```python
from build123d import *

# Parameters (mm, degrees)
PAD005_DEPTH    = 2
SKETCH011_W     = 2
SKETCH011_H     = 6
PAD006_DEPTH    = 2
PAD006_FACE12_W = 2
PAD006_FACE12_H = 6
PAD007_DEPTH    = 2
PAD007_FACE15_W = 2
PAD007_FACE15_H = 6
PAD008_DEPTH    = 2
FILLET_R        = 1
SKETCH012_R     = 0.75
SKETCH012_W     = 12.5
SKETCH012_H     = 24
POCKET004_DEPTH = 5


with BuildPart() as part:
    # Sketch009 → Pad005 (new body)
    with BuildSketch(Plane(origin=(0, 32.75, 0), x_dir=(-1, 0, 0), z_dir=(0, 1, 0))):
        Polygon((13, 24.5), (-13, 24.5), (-13, -24.5), (13, -24.5), (13, -2.75), (15.4, -2.75), (15.4, 2.75), (13, 2.75), align=None)
    extrude(amount=PAD005_DEPTH)

    # Sketch011 (on Face9 of Pad005) → Pad006 (join)
    with BuildSketch(Plane.XZ.offset(-32.75)):
        with Locations((11.5, 15)):
            Rectangle(SKETCH011_W, SKETCH011_H)
        with Locations((11.5, -15)):
            Rectangle(SKETCH011_W, SKETCH011_H)
    extrude(amount=PAD006_DEPTH)

    # Pad006 Face12 → Pad007 (add)
    with BuildSketch(Plane(origin=(12.5, 31.75, 15), x_dir=(0, -1, 0), z_dir=(1, 0, 0))):
        Rectangle(PAD006_FACE12_W, PAD006_FACE12_H)
    extrude(amount=PAD007_DEPTH)

    # Pad007 Face15 → Pad008 (add)
    with BuildSketch(Plane(origin=(12.5, 31.75, -15), x_dir=(0, -1, 0), z_dir=(1, 0, 0))):
        Rectangle(PAD007_FACE15_W, PAD007_FACE15_H)
    extrude(amount=PAD008_DEPTH)

    # Fillet
    fillet_edges = [part.edges().sort_by_distance(p)[0] for p in [
        (14.5, 30.75, -15),
        (14.5, 30.75, 15),
        (10.5, 30.75, 15),
        (10.5, 30.75, -15),
        (12.5, 30.75, 18),
        (12.5, 30.75, 12),
        (12.5, 30.75, -12),
        (12.5, 30.75, -18),
    ]]
    fillet(fillet_edges, radius=FILLET_R)

    # Sketch012 (on Face23 of Fillet) → Pocket004 (cut)
    with BuildSketch(Plane(origin=(0, 34.75, 0), x_dir=(1, 0, 0), z_dir=(0, 1, 0))):
        with Locations((0, 13.5)):
            Circle(SKETCH012_R)
        with Locations((0, -13.5)):
            Circle(SKETCH012_R)
        Rectangle(SKETCH012_W, SKETCH012_H)
    extrude(amount=-POCKET004_DEPTH, mode=Mode.SUBTRACT)


solid = part.part
```
Input: part model. Units: mm. Frame: model coordinates. A direction names the side the tool comes from. Coordinates: 2 decimals unless noted, no trailing zeros. Order: outer loops, then holes, each group sorted by start corner. A loop starts at its lowest first (then second) coordinate and runs counter-clockwise, first axis right, second up. Notation, with made-up numbers: (32.5, -17.5) - (38.5, -17.5) arc R24 ccw to (38.5, 18.5) - close; hole circle Ø2 at (33.25, -39.75). An arc over 180 degrees is marked (long way). Return JSON: item names as keys, results as strings.
Q1. Cut plane C-C (x = 0). Return loops of the section in (y, z), then the cut area to 3 significant figures.
The answers:
{"outline": "(32.75, -24.5) - (34.75, -24.5) - (34.75, -14.25) - (32.75, -14.25) - close; (32.75, -12.75) - (34.75, -12.75) - (34.75, -12) - (32.75, -12) - close; (32.75, 12) - (34.75, 12) - (34.75, 12.75) - (32.75, 12.75) - close; (32.75, 14.25) - (34.75, 14.25) - (34.75, 24.5) - (32.75, 24.5) - close", "area": "44.0 mm2"}
Q2. Cut plane D-D (z = -13.5). Return loops of the section in (x, y), then the cut area to 3 significant figures.
The answers:
{"outline": "(-13, 32.75) - (-0.75, 32.75) - (-0.75, 34.75) - (-13, 34.75) - close; (0.75, 32.75) - (10.5, 32.75) - (10.5, 31.75) arc R1 ccw to (11.5, 30.75) - (13.5, 30.75) arc R1 ccw to (14.5, 31.75) - (14.5, 32.75) - (13, 32.75) - (13, 34.75) - (0.75, 34.75) - close", "area": "56.6 mm2"}
Q3. Draft query along X for faces 1 (the cylindrical face through (-0.098, 33.764, 12.756)), 2 (the flat face through (14.5, 32, -15)), 3 (the flat face through (-7, 34.75, 0)), 4 (the flat face through (-15.4, 34, 0)). Return one class per face: +X half, -X half, draft (parallel to the pull), parting line (faces both ways), or undercut.
The answers:
{"face 1": "undercut", "face 2": "+X half", "face 3": "draft", "face 4": "-X half"}
Q4. Cut plane A-A (z = 7). Return loops of the section in (x, y).
The answers:
{"outline": "(-13, 32.75) - (-6.25, 32.75) - (-6.25, 34.75) - (-13, 34.75) - close; (6.25, 32.75) - (13, 32.75) - (13, 34.75) - (6.25, 34.75) - close"}
Q5. Ray query, probe 1 along Z at (x, y) = (0, 33.3); probe 2 along X at (y, z) = (33.8, 13.5); probe 3 along Z at (x, y) = (4, 34.4). Return the intervals inside material, ascending.
The answers:
{"probe 1": "z = -24.5 to -14.25, -12.75 to -12, 12 to 12.75, 14.25 to 24.5", "probe 2": "x = -13 to -0.75, 0.75 to 13", "probe 3": "z = -24.5 to -12, 12 to 24.5"}
Q6. First-contact query: pin 1 (0.6 mm diameter, centred on x = -14.5, y = 33.5, fed in from -Z); pin 2 (0.8 mm diameter, centred on x = 13.5, z = 15.5, fed in from +Y); pin 3 (1 mm diameter, centred on y = 34, z = -11, fed in from -X). Flat tips, straight axial feed; report the tip coordinate or a pass-through.
The answers:
{"pin 1": "stops at z = -2.75", "pin 2": "stops at y = 32.75", "pin 3": "stops at x = -13"}
Q7. Cut plane B-B (y = 33.7). Return loops of the section in (x, z), then the cut area to 3 significant figures.
The answers:
{"outline": "(-15.4, -2.75) - (-13, -2.75) - (-13, -24.5) - (13, -24.5) - (13, 24.5) - (-13, 24.5) - (-13, 2.75) - (-15.4, 2.75) - close; hole (-6.25, -12) - (6.25, -12) - (6.25, 12) - (-6.25, 12) - close; hole circle Ø1.5 at (0, -13.5); hole circle Ø1.5 at (0, 13.5)", "area": "984 mm2"}
Q8. Access query for faces 5 (the flat face through (-14, 34, 2.75)), 6 (the flat face through (12, 32, -18)), 7 (the flat face through (12, 32, 18)), 8 (the cylindrical face through (12.47, 31.19, 12.17)). Directions: +Z, -Z, +X, -X, +Y, -Y. A direction counts if a zero-diameter tool reaches every point of the face in a straight line with its end or side. Return the directions, or none.
The answers:
{"face 5": "+Z, -X, +Y, -Y", "face 6": "-Z, +X, -X, -Y", "face 7": "+Z, +X, -X, -Y", "face 8": "+X, -X, -Y"}
